Geometry: see drawing. Coordinates: mm, zero at the bounding-box minimum. A direction names the side the tool comes from. Give positions to 0.01 mm unless a question says otherwise; leave off trailing zeros. Write each loop counter-clockwise with the first axis right and the second up, starting at its lowest first coordinate (ties: lowest second). Pieces come first, ordered by that corner, then holes. Notation, with made-up numbers: (14, 41) -> (39, 41) arc R32 ccw to (39, 71) -> close; hole circle Ø1 at (-22.75, 85.25). An arc over 180 degrees is marked (long way). Use CSV: the item, a comma, the result in double quotes. Start each with the question number.
1) Section D-D (y = 4). Output: boundary loops of the cut face in (x, z).
2) Section A-A (x = 108). Output: boundary loops of the cut face in (y, z), plus the area to 3 significant figures.
3) Set-up query: the marked faces 1, 2 and 3. Return all of +Z, -Z, +X, -X, +Y, -Y with unobstructed straight access to the full face (end or side cutting, diameter ignored); none if empty.
4) Draft query along X for the marked faces 4, 5 and 6. Return one class per face: pulls with the +X half, pulls with the -X half, needs draft (parallel to the pull), parting line crosses it, or undercut.
5) Section B-B (y = 19.5). Output: boundary loops of the cut face in (x, z).
6) Contact query for flat-ended pins moving along their axis: P1, Ø18.5, axis at y = 21, z = 24, coming from the -X side; P2, Ø6.5, axis at x = 14.5, y = 16, coming from the -Z side; P3, Ø9, axis at y = 6, z = 18, coming from the -X side; P4, Ø6, axis at x = 58, z = 12.5, coming from the +Y side. Output: stop coordinate, or through.
7) Material intervals for line 1 (X direction, y = 25, z = 34.5); line 2 (Y direction, x = 121, z = 25); line 3 (Y direction, x = 65.5, z = 12), sorted ascending. Write a range as [from, to].
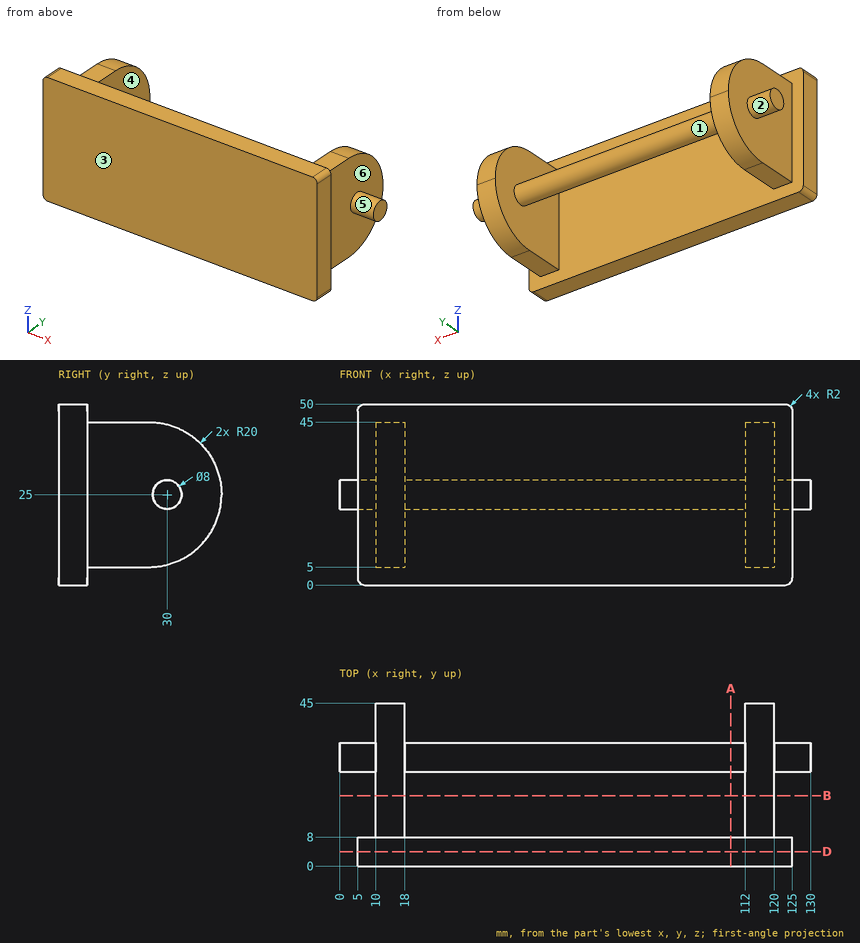
Answers follow:
1,outline,"(5, 2) arc R2 ccw to (7, 0) -> (123, 0) arc R2 ccw to (125, 2) -> (125, 48) arc R2 ccw to (123, 50) -> (7, 50) arc R2 ccw to (5, 48) -> close"
2,outline,"(0, 0) -> (8, 0) -> (8, 50) -> (0, 50) -> close; circle Ø8 at (30, 25)"
2,area,"450 mm^2"
3,face 1,"none"
3,face 2,"-X"
3,face 3,"+Z, -Z, +X, -X, -Y"
4,face 4,"undercut"
4,face 5,"needs draft"
4,face 6,"pulls with the +X half"
5,outline,"(10, 5) -> (18, 5) -> (18, 45) -> (10, 45) -> close; (112, 5) -> (120, 5) -> (120, 45) -> (112, 45) -> close"
6,P1,"stops at x = 0"
6,P2,"stops at z = 5"
6,P3,"stops at x = 5"
6,P4,"stops at y = 8"
7,line 1,"x = [10, 18], [112, 120]"
7,line 2,"y = [0, 8], [26, 34]"
7,line 3,"y = [0, 8]"
